For this review, use the dimensioned drawing (mm, ordinates from the lowest corner) and the shaded views. Coordinates: 2 decimals unless noted, no trailing zeros. Write each loop counter-clockwise with the first axis right and the second up, starting at its lowest first coordinate (ties: lowest second). Pieces come first, ordered by that corner, then holes. Notation, with made-up numbers: (-4.75, 31.25) - (33.25, 31.25) arc R32 cw to (33.25, 61.25) - close; hole circle Ø6 at (-35.75, 48.5). An arc over 180 degrees is marked (long way). Answer as a JSON object with one key per item and string values.
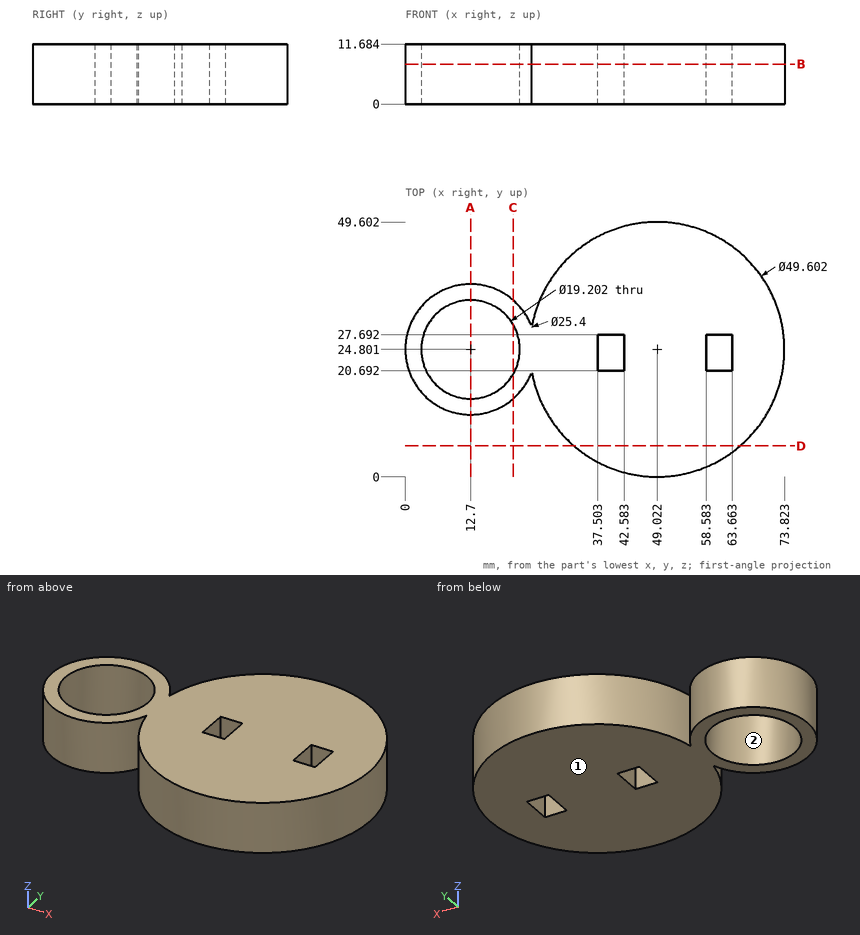
(1) Take a section at B-B, the plane z = 7.75. Write out the cut boundary in (x, y), and give its area (3 significant figures).
Solved:
{"outline": "(24.61, 20.4) arc R24.8 ccw (long way) to (24.61, 29.2) arc R12.7 ccw (long way) to start; hole circle Ø19.2 at (12.7, 24.8); hole (37.5, 20.69) - (42.58, 20.69) - (42.58, 27.69) - (37.5, 27.69) - close; hole (58.58, 20.69) - (63.66, 20.69) - (63.66, 27.69) - (58.58, 27.69) - close", "area": "2,070 mm^2"}
(2) To check wall thickness, follow line 1 (Y direction, x = 12.7, z = 5.25); line 2 (X direction, y = 21.5, z = 7.75) (1 decimal); line 3 (Y direction, x = 11.5, z = 5.75) (1 decimal). State the ranges of each line that lie inside material, in increasing order. Write a range as from..to.
Solved:
{"line 1": "y = 12.1..15.2, 34.4..37.5", "line 2": "x = 0.4..3.7, 21.7..37.5, 42.6..58.6, 63.7..73.6", "line 3": "y = 12.2..15.3, 34.3..37.4"}
(3) The part is to be moulded in two halves that separate along Y. For the marked faces 1 and 2, say which applies: pulls with the +Y half, pulls with the -Y half, needs draft (parallel to the pull), parting line crosses it, or undercut.
Solved:
{"face 1": "needs draft", "face 2": "undercut"}
(4) Take a section at D-D, the plane y = 6. Write out the cut boundary in (x, z), and give its area (3 significant figures).
Solved:
{"outline": "(32.85, 0) - (65.2, 0) - (65.2, 11.68) - (32.85, 11.68) - close", "area": "378 mm^2"}
(5) Take a section at A-A, the plane x = 12.7. Write out the cut boundary in (y, z).
Solved:
{"outline": "(12.1, 0) - (15.2, 0) - (15.2, 11.68) - (12.1, 11.68) - close; (34.4, 0) - (37.5, 0) - (37.5, 11.68) - (34.4, 11.68) - close"}
(6) For pin 1 (4 mm diameter, centred on x = 41.5, z = 4.5, fed in from +Y); pin 2 (1.5 mm diameter, centred on x = 26.5, z = 4.5, fed in from -Y) (1 decimal); pin 3 (2 mm diameter, centred on x = 63.5, z = 10, fed in from +Y), all flat-tipped, find the tip position at first contact; note any pin that passes through.
Solved:
{"pin 1": "stops at y = 48.98", "pin 2": "stops at y = 12.9", "pin 3": "stops at y = 45.62"}
(7) Take a section at C-C, the plane x = 21. Write out the cut boundary in (y, z) (1 decimal), and give its area (3 significant figures).
Solved:
{"outline": "(15.2, 0) - (20, 0) - (20, 11.7) - (15.2, 11.7) - close; (29.6, 0) - (34.4, 0) - (34.4, 11.7) - (29.6, 11.7) - close", "area": "112 mm^2"}
